Check sheet for the modelled part. Datum: model origin and axes. Units: mm. Face numbers are marked on the shaded views. A direction names the side the tool comes from. Give positions to 0.01 mm unless a question says otherwise; leave off trailing zeros. Write each loop counter-clockwise with the first axis right and the second up, starting at its lowest first coordinate (ties: lowest second). Pieces come first, ordered by that corner, then holes.
from build123d import *

# Parameters (mm, degrees)
SKETCH1_R           = 42.5
BOSS_EXTRUDE1_DEPTH = 2.5
SKETCH3_W           = 13
SKETCH3_H           = 18
BOSS_EXTRUDE2_DEPTH = 20
SKETCH4_R           = 8.9
CUT_EXTRUDE2_DEPTH  = 20
SKETCH5_R           = 8.9
CUT_EXTRUDE3_DEPTH  = 20
SKETCH6_R           = 8.9
CUT_EXTRUDE4_DEPTH  = 20
CUT_EXTRUDE5_START  = -20
SKETCH7_R           = 8.9
CUT_EXTRUDE5_DEPTH  = 20
CUT_EXTRUDE6_START  = -20
SKETCH8_R           = 8.9
CUT_EXTRUDE6_DEPTH  = 20
CUT_EXTRUDE7_START  = -20
SKETCH9_R           = 8.9
CUT_EXTRUDE7_DEPTH  = 20
CUT_EXTRUDE8_DEPTH  = 76.388
SKETCH11_W          = 71.811217628
SKETCH11_H          = 11.984599711
CUT_EXTRUDE9_DEPTH  = 76.388
SKETCH12_R          = 18.204170311
CUT_EXTRUDE10_DEPTH = 76.388
SKETCH13_R          = 1.997627935
CUT_EXTRUDE11_DEPTH = 10


with BuildPart() as part:
    # Sketch1 → Boss-Extrude1 (new body)
    with BuildSketch(Plane(origin=(0, 0, 0), x_dir=(1, 0, 0), z_dir=(0, 1, 0))):
        with Locations(Location((0, 0, 0), (0, 0, 270))):
            Circle(SKETCH1_R)
    extrude(amount=BOSS_EXTRUDE1_DEPTH)

    # Sketch3 → Boss-Extrude2 (add)
    with BuildSketch(Plane(origin=(0, 2.5, 0), x_dir=(1, 0, 0), z_dir=(0, 1, 0))):
        with Locations((-26.394376419, 0)):
            Rectangle(SKETCH3_W, SKETCH3_H)
        with Locations((26.394376419, 0)):
            Rectangle(SKETCH3_W, SKETCH3_H)
        Polygon((-8.599367677, 32.894541729), (-2.099367677, 21.63621148), (-17.687824945, 12.63621148), (-24.187824945, 23.894541729), align=None)
        Polygon((8.599367677, 32.894541729), (24.187824945, 23.894541729), (17.687824945, 12.63621148), (2.099367677, 21.63621148), align=None)
        Polygon((8.599367677, -32.894541729), (2.099367677, -21.63621148), (17.687824945, -12.63621148), (24.187824945, -23.894541729), align=None)
        Polygon((-8.599367677, -32.894541729), (-24.187824945, -23.894541729), (-17.687824945, -12.63621148), (-2.099367677, -21.63621148), align=None)
    extrude(amount=BOSS_EXTRUDE2_DEPTH)

    # Sketch4 → Cut-Extrude2 (cut)
    with BuildSketch(Plane.ZY.offset(32.894376419)):
        with Locations((0, 12.5)):
            Circle(SKETCH4_R)
    extrude(amount=-CUT_EXTRUDE2_DEPTH, mode=Mode.SUBTRACT)

    # Sketch5 → Cut-Extrude3 (cut)
    with BuildSketch(Plane(origin=(-16.393596311, 0, 28.394541729), x_dir=(0.8660254037844386, 0, 0.5000000000000003), z_dir=(-0.5000000000000003, 0, 0.8660254037844386))):
        with Locations((0, 12.5)):
            Circle(SKETCH5_R)
    extrude(amount=-CUT_EXTRUDE3_DEPTH, mode=Mode.SUBTRACT)

    # Sketch6 → Cut-Extrude4 (cut)
    with BuildSketch(Plane(origin=(16.393596311, 0, 28.394541729), x_dir=(0.8660254037844386, 0, -0.5000000000000003), z_dir=(0.5000000000000003, 0, 0.8660254037844386))):
        with Locations((0, 12.5)):
            Circle(SKETCH6_R)
    extrude(amount=-CUT_EXTRUDE4_DEPTH, mode=Mode.SUBTRACT)

    # Sketch7 → Cut-Extrude5 (cut)
    with BuildSketch(Plane(origin=(32.894376419, 0, 0), x_dir=(0, 0, -1), z_dir=(1, 0, 0)).offset(CUT_EXTRUDE5_START)):
        with Locations(Location((0, 12.5, 0), (0, 0, 180))):
            Circle(SKETCH7_R)
    extrude(amount=CUT_EXTRUDE5_DEPTH, mode=Mode.SUBTRACT)

    # Sketch8 → Cut-Extrude6 (cut)
    with BuildSketch(Plane(origin=(16.393596311, 0, -28.394541729), x_dir=(-0.8660254037844386, 0, -0.5000000000000003), z_dir=(0.5000000000000003, 0, -0.8660254037844386)).offset(CUT_EXTRUDE6_START)):
        with Locations(Location((0, 12.5, 0), (0, 0, 180))):
            Circle(SKETCH8_R)
    extrude(amount=CUT_EXTRUDE6_DEPTH, mode=Mode.SUBTRACT)

    # Sketch9 → Cut-Extrude7 (cut)
    with BuildSketch(Plane(origin=(-16.393596311, 0, -28.394541729), x_dir=(-0.8660254037844386, 0, 0.5000000000000003), z_dir=(-0.5000000000000003, 0, -0.8660254037844386)).offset(CUT_EXTRUDE7_START)):
        with Locations(Location((0, 12.5, 0), (0, 0, 180))):
            Circle(SKETCH9_R)
    extrude(amount=CUT_EXTRUDE7_DEPTH, mode=Mode.SUBTRACT)

    # Sketch10 → Cut-Extrude8 (cut)
    with BuildSketch(Plane(origin=(-16.393596311, 0, -28.394541729), x_dir=(-0.8660254037844386, 0, 0.5000000000000003), z_dir=(-0.5000000000000003, 0, -0.8660254037844386))):
        Polygon((-35.669118209, 18.214643823), (-9, 18.214643823), (-9, 22.5), (-6.822964603, 22.5), (-6.822964603, 25.559573076), (-35.669118209, 25.559573076), align=None)
        Polygon((-6.822964603, 25.559573076), (-6.822964603, 22.5), (9, 22.5), (9, 18.214643823), (33.747549551, 18.214643823), (33.747549551, 25.559573076), align=None)
    extrude(amount=-CUT_EXTRUDE8_DEPTH, mode=Mode.SUBTRACT)

    # Sketch11 → Cut-Extrude9 (cut)
    with BuildSketch(Plane(origin=(-16.393596311, 0, -28.394541729), x_dir=(-0.8660254037844386, 0, 0.5000000000000003), z_dir=(-0.5000000000000003, 0, -0.8660254037844386))):
        with Locations((1.515702587, 16.507700144)):
            Rectangle(SKETCH11_W, SKETCH11_H)
    extrude(amount=-CUT_EXTRUDE9_DEPTH, mode=Mode.SUBTRACT)

    # Sketch12 → Cut-Extrude10 (cut)
    with BuildSketch(Plane(origin=(0, 2.5, 0), x_dir=(1, 0, 0), z_dir=(0, 1, 0))):
        with Locations(Location((0, 0, 0), (0, 0, 270))):
            Circle(SKETCH12_R)
    extrude(amount=-CUT_EXTRUDE10_DEPTH, mode=Mode.SUBTRACT)

    # Sketch13 → Cut-Extrude11 (cut)
    with BuildSketch(Plane(origin=(0, 2.5, 0), x_dir=(1, 0, 0), z_dir=(0, 1, 0))):
        with Locations(Location((-22.072556502, 12.515367089, 0), (0, 0, 270))):
            Circle(SKETCH13_R)
        with Locations(Location((22.072556502, 12.515367089, 0), (0, 0, 270))):
            Circle(SKETCH13_R)
        with Locations(Location((22.072556502, -12.515367089, 0), (0, 0, 270))):
            Circle(SKETCH13_R)
        with Locations(Location((-22.072556502, -12.515367089, 0), (0, 0, 270))):
            Circle(SKETCH13_R)
    extrude(amount=-CUT_EXTRUDE11_DEPTH, mode=Mode.SUBTRACT)


solid = part.part
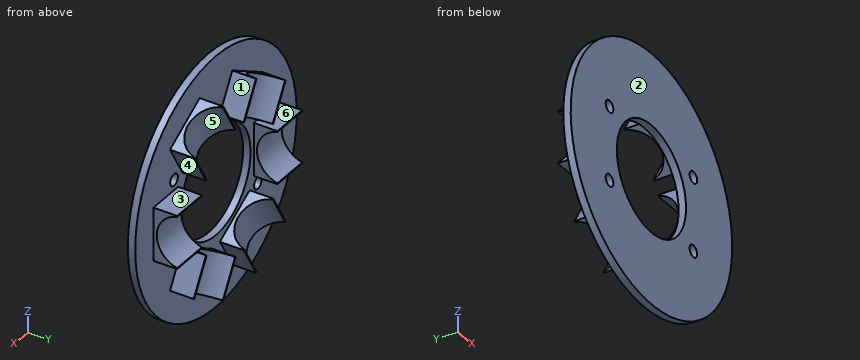
1) Sectioned sample at A-A on x = 0. Record the boundary of the cut face in (y, z), then the cut area to 3 significant figures.
2) Access from +Z, -Z, +X, -X, +Y, -Y to the whole of each face (thin tool, end or side, straight path). Record for the marked faces 4, 5 and 6.
3) Gauge pin test, flat ends, axial feed: pin 1 (2.5 mm diameter, centred on y = 5.5, z = 0.5, fed in from -X); pin 2 (5 mm diameter, centred on x = 16.5, z = 29, fed in from +Y); pin 3 (10 mm diameter, centred on x = -9.5, z = 18.5, fed in from +Y); pin 4 (4.5 mm diameter, centred on x = -22.07, z = -12.52, fed in from +Y). Record the tip position at first contact, or that the pin passes through.
4) Sectioned sample at D-D on y = 6.25. Give the number of separate pieces and of enclosed holes in the cut face, then the cut area to 3 significant figures.
5) Sectioned sample at B-B on z = 0. Record the boundary of the cut face in (x, y), then the cut area to 3 significant figures.
6) Draft check along Z on the marked faces 1, 2 and 3. Enter one of: +Z half, -Z half, draft (parallel to the pull), parting line (faces both ways), or undercut.
7) Scan lines: L1, parallel to Z at x = 23, y = 6.25; L2, parallel to Y at x = -3, z = 36; L3, parallel to X at y = 3.75, z = -8.5. Record each from-to range of solid material in increasing order.
8) Sectioned sample at C-C on y = 1.25. Record the boundary of the cut face in (x, z), then the cut area to 3 significant figures.
Answers below:
1. outline: (0, -42.5) - (2.5, -42.5) - (2.5, -18.2) - (0, -18.2) - close; (0, 18.2) - (2.5, 18.2) - (2.5, 42.5) - (0, 42.5) - close
1. area: 121 mm2
2. face 4: +X, +Y
2. face 5: +Y
2. face 6: +X, -X, +Y
3. pin 1: passes through
3. pin 2: stops at y = 4
3. pin 3: stops at y = 5.95
3. pin 4: stops at y = 2.5
4. separate pieces: 12
4. enclosed holes: 0
4. area: 416 mm2
5. outline: (-42.5, 0) - (-18.2, 0) - (-18.2, 2.5) - (-19.89, 2.5) - (-19.89, 3.6) - (-32.89, 3.6) - (-32.89, 2.5) - (-42.5, 2.5) - close; (18.2, 0) - (42.5, 0) - (42.5, 2.5) - (32.89, 2.5) - (32.89, 3.6) - (19.89, 3.6) - (19.89, 2.5) - (18.2, 2.5) - close
5. area: 150 mm2
6. face 1: +Z half
6. face 2: draft
6. face 3: undercut
7. L1: z = -24.58 to -21.84, -9 to -6.34, 6.34 to 9, 21.84 to 24.58
7. L2: y = 0 to 2.5
7. L3: x = -32.89 to -19.89, 19.89 to 32.89
8. outline: circle Ø85 at (0, 0); hole circle Ø4 at (-22.07, -12.52); hole circle Ø4 at (-22.07, 12.52); hole circle Ø36.41 at (0, 0); hole circle Ø4 at (22.07, -12.52); hole circle Ø4 at (22.07, 12.52)
8. area: 4,580 mm2
